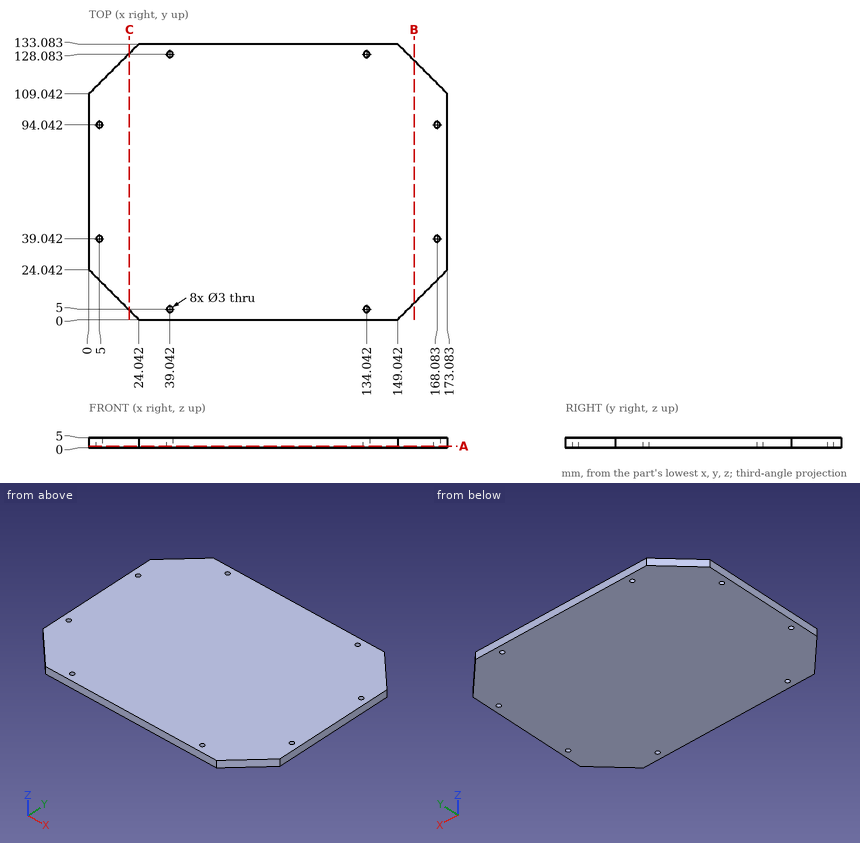
Could you check a few things on this drawing? It's one solid part, dimensions in mm from its lowest x, y, z. Coordinates: 2 decimals unless noted, no trailing zeros. Order: outer loops, then holes, each group sorted by start corner. A loop starts at its lowest first (then second) coordinate and runs counter-clockwise, first axis right, second up. Notation, with made-up numbers: M 52,78.5 L 76,78.5 A10 ccw 76,85.5 Z; hole C 88,80 d3. An arc over 180 degrees is marked long. Use a Markdown table: item, result. Add a question column.
Q1. I want a section at B-B on x = 157. List the corners of the cut face in (y, z) for me (1 decimal).
Q2. I want a section at C-C on x = 19.5. List the corners of the cut face in (y, z) for me, then the cut area to 3 significant figures.
Q3. I'm going to push a flat-ended pin straight in: pin 1 (3 mm diameter, centred on y = 15, z = 3.5, fed in from -X). Where does the tip first touch, or does it pass through?
Q4. If I drill on L1, parallel to Y at x = 20.5, z = 2.45; L2, parallel to Y at x = 153.5, z = 1.3 (1 decimal); L3, parallel to X at y = 125, z = 3.6 (1 decimal), over which ranges is the centre line in solid material (lowest first)?
Q5. I want a section at A-A on z = 0.85. Give the number of separate pieces and of enclosed holes in the cut face, then the cut area to 3 significant figures.
Checked values:
| question | item | result |
|---|---|---|
| 1 | outline | M 8,0 L 125.1,0 L 125.1,5 L 8,5 Z |
| 2 | outline | M 4.54,0 L 128.54,0 L 128.54,5 L 4.54,5 Z |
| 2 | area | 620 mm² |
| 3 | pin 1 | x = 7.54 |
| 4 | L1 | 3.54 to 129.54 |
| 4 | L2 | 4.5 to 128.6 |
| 4 | L3 | 16 to 157.1 |
| 5 | separate pieces | 1 |
| 5 | enclosed holes | 8 |
| 5 | area | 21,800 mm² |
